Here's how the part is built. I have some questions about the finished solid (model axes, mm). Face numbers are marked on the shaded views. A direction names the side the tool comes from. Coordinates: 2 decimals unless noted, no trailing zeros. Loops run counter-clockwise (first coordinate to the right, second up) from the corner with the lowest first, then second, coordinate; pieces in that order, holes last. Notation, with made-up numbers: M 69.5,17 L 109.5,17 A31 ccw 109.5,42 Z; hole C 6,27.5 d10. An arc over 180 degrees is marked long. Use one line per item in the form item = value. Start each with the question number.
(1) Imagine slicing it at C-C, the plane z = 1.25. Please give me the cut outline in (x, y), and give its area (3 significant figures).
(2) Thinking about a two-plate mould opening in X: for the marked faces 1, 2 and 3, which applies, +X half, -X half, draft (parallel to the pull), parting line (faces both ways), or undercut?
(3) Please list where these lines run through material, in increasing order: L1, parallel to Y at x = 0, z = 4.5; L2, parallel to Y at x = 0, z = 3.25; L3, parallel to Y at x = 5, z = 2.5.
(4) Imagine slicing it at D-D, the plane x = -12. Please give me the cut outline in (y, z).
(5) Imagine slicing it at A-A, the plane y = 0. Please give me the cut outline in (x, z).
(6) Will these pins go through, and if not, where does the flat tip stop? P1, Ø1.3, axis at x = -10.5, z = 2.5, coming from the +Y side; P2, Ø1.5, axis at x = 13.5, y = 7.5, coming from the +Z side; P3, Ø3.5, axis at y = 7.5, z = 2.5, coming from the -X side.
(7) On a 3-axis mill with a long thin cutter (end or side, diameter ignored), from which of +Z, -Z, +X, -X, +Y, -Y can I reach the whole of each face in a straight line? I mean the marked faces 4, 5 and 6. Say none if no direction works.
```python
from build123d import *

# Parameters (mm, degrees)
F0_R     = 15
F1_DEPTH = 4
F2_R     = 18
F2_R_2   = 15
F3_DEPTH = 0.5
F4_R     = 4
F5_DEPTH = 3
F6_R     = 1.55
F7_DEPTH = 7.5
F9_DEPTH = 4.5


with BuildPart() as f1:
    # F0 (on Top) → F1 (new body)
    with BuildSketch(Plane.XY):
        Circle(F0_R)
    extrude(amount=F1_DEPTH)

    # F2 (on face) → F3 (join)
    with BuildSketch(Plane(origin=(0, 0, 0), x_dir=(1, 0, 0), z_dir=(0, 0, -1))):
        Circle(F2_R)
        Circle(F2_R_2, mode=Mode.SUBTRACT)
        Circle(F2_R_2)
    extrude(amount=F3_DEPTH)

    # F4 (on face) → F5 (join)
    with BuildSketch(Plane.XY.offset(4)):
        Circle(F4_R)
    extrude(amount=F5_DEPTH)

    # F6 (on face) → F7 (cut, through all)
    with BuildSketch(Plane.XY.offset(7)):
        Circle(F6_R)
    extrude(amount=-F7_DEPTH, mode=Mode.SUBTRACT)

    # F8 (on face) → F9 (cut, through all)
    with BuildSketch(Plane.XY.offset(4)):
        with BuildLine():
            ThreePointArc((-5.4083269132, 1), (-3.8890872965, 3.8890872965), (-1, 5.4083269132))
            Line((-1, 5.4083269132), (-1, 13.4629120178))
            ThreePointArc((-1, 13.4629120178), (-9.545941546, 9.545941546), (-13.4629120178, 1))
            Line((-13.4629120178, 1), (-5.4083269132, 1))
        make_face()
        with BuildLine():
            Line((1, 13.4629120178), (1, 5.4083269132))
            ThreePointArc((1, 5.4083269132), (3.8890872965, 3.8890872965), (5.4083269132, 1))
            Line((5.4083269132, 1), (13.4629120178, 1))
            ThreePointArc((13.4629120178, 1), (9.545941546, 9.545941546), (1, 13.4629120178))
        make_face()
        with BuildLine():
            Line((13.4629120178, -1), (5.4083269132, -1))
            ThreePointArc((5.4083269132, -1), (3.8890872965, -3.8890872965), (1, -5.4083269132))
            Line((1, -5.4083269132), (1, -13.4629120178))
            ThreePointArc((1, -13.4629120178), (9.545941546, -9.545941546), (13.4629120178, -1))
        make_face()
        with BuildLine():
            ThreePointArc((-1, -5.4083269132), (-3.8890872965, -3.8890872965), (-5.4083269132, -1))
            Line((-5.4083269132, -1), (-13.4629120178, -1))
            ThreePointArc((-13.4629120178, -1), (-9.545941546, -9.545941546), (-1, -13.4629120178))
            Line((-1, -13.4629120178), (-1, -5.4083269132))
        make_face()
    extrude(amount=-F9_DEPTH, mode=Mode.SUBTRACT)


solid = f1.part
```
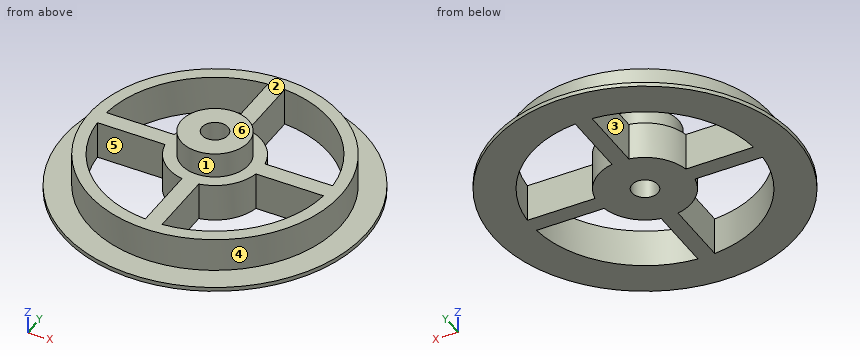
Answer:
q1.outline = C 0,0 d30; hole M -13.46,-1 A13.5 ccw -1,-13.46 L -1,-5.41 A5.5 cw -5.41,-1 Z; hole M -13.46,1 L -5.41,1 A5.5 cw -1,5.41 L -1,13.46 A13.5 ccw Z; hole C 0,0 d3.1; hole M 1,-13.46 A13.5 ccw 13.46,-1 L 5.41,-1 A5.5 cw 1,-5.41 Z; hole M 1,5.41 A5.5 cw 5.41,1 L 13.46,1 A13.5 ccw 1,13.46 Z
q1.area = 286 mm²
q2.face_1 = parting line
q2.face_2 = draft
q2.face_3 = undercut
q3.L1 = -4 to -1.55, 1.55 to 4
q3.L2 = -15 to -1.55, 1.55 to 15
q3.L3 = -14.14 to -12.54, -2.29 to 2.29, 12.54 to 14.14
q4.outline = M -13.42,-0.5 L -6.18,-0.5 L -6.18,4 L -9,4 L -9,0 L -13.42,0 Z; M -1,-0.5 L 1,-0.5 L 1,4 L -1,4 Z; M 6.18,-0.5 L 13.42,-0.5 L 13.42,0 L 9,0 L 9,4 L 6.18,4 Z
q5.outline = M -18,-0.5 L -1.55,-0.5 L -1.55,7 L -4,7 L -4,4 L -15,4 L -15,0 L -18,0 Z; M 1.55,-0.5 L 18,-0.5 L 18,0 L 15,0 L 15,4 L 4,4 L 4,7 L 1.55,7 Z
q6.P1 = 11.31
q6.P2 = 4
q6.P3 = -13.85
q7.face_4 = +Z
q7.face_5 = +Z, -Z
q7.face_6 = +Z, +X, -X, +Y, -Y
